from build123d import *

# Parameters (mm, degrees)
F0_W     = 17.78
F0_H     = 101.6
F0_R     = 2.794
F1_DEPTH = 5.08
F2_W     = 17.78
F2_H     = 12.7
F3_DEPTH = 19.05


with BuildPart() as f1:
    # F0 (on Top) → F1 (new body)
    with BuildSketch(Plane.XY):
        with Locations((0, 12.7)):
            Rectangle(F0_W, F0_H)
        with Locations((0, -30.513791)):
            Circle(F0_R, mode=Mode.SUBTRACT)
        with Locations((0, 20.286209)):
            Circle(F0_R, mode=Mode.SUBTRACT)
    extrude(amount=F1_DEPTH)

    # F2 (on face) → F3 (join)
    with BuildSketch(Plane.XY.offset(5.08)):
        with Locations((0, 57.15)):
            Rectangle(F2_W, F2_H)
    extrude(amount=F3_DEPTH)


solid = f1.part
Can you work these out from the model? Positions are in its coordinate system, mm. A direction names the side the tool comes from. Coordinates: 2 decimals unless noted, no trailing zeros. Write each loop counter-clockwise with the first axis right and the second up, starting at its lowest first coordinate (ties: lowest second). Pieces come first, ordered by that corner, then holes. Notation, with made-up numbers: (18, 73.25) - (58, 73.25) arc R18 cw to (58, 95.25) - close; hole circle Ø8 at (28.5, -21). An arc over 180 degrees is marked (long way). Return JSON: item names as keys, results as strings. Group by question number.
Item 1: Which directions (+Z, -Z, +X, -X, +Y, -Y) give clear straight access to the entire face, cutting with the end or side of a thin tool? Please do faces 5 (the face through (0, 7, 5.08)), 6 (the face through (-8.89, 24, 3)).
Item 2: If we section it at A-A (x = 0): Write out the boundary of the cut face in (y, z).
Item 3: I'm going to push flat-ended pins straight in: pin 1 Ø6 at (x, y) = (5.5, 28.5) entering from -Z; pin 2 Ø9 at (x, z) = (-0.5, 17) entering from -Y; pin 3 Ø3 at (x, y) = (-3, -13) entering from +Z. Where does each tip first touch, or does it pass through?
Item 4: If we section it at D-D (z = 9.5): Write out the boundary of the cut face in (x, y).
Item 5: We'd pull the mould along Y, two halves only. Please class faces 1 (the face through (0, 63.5, 12)), 2 (the face through (0, 57, 24.13)), 3 (the face through (-0.364, 23.056, 2.504)), 4 (the face through (-0.61, -33.24, 2.5)): pulls with the +Y half, pulls with the -Y half, needs draft (parallel to the pull), parting line crosses it, or undercut.
Item 6: If we section it at C-C (x = -7.5): Write out the boundary of the cut face in (y, z).
Item 7: If we section it at B-B (y = 19): Write out the boundary of the cut face in (x, z).
Item 8: Please list where these lines run through material, in increasing order: probe 1 along Y at (x, z) = (0, 4); probe 2 along Y at (x, z) = (-1.25, 3.5) (3 decimals); probe 3 along Y at (x, z) = (-6, 14.5).
Return value:
{
 "1": {"face 5": "+Z, +X, -X, -Y", "face 6": "+Z, -Z, -X, +Y, -Y"},
 "2": {"outline": "(-38.1, 0) - (-33.31, 0) - (-33.31, 5.08) - (-38.1, 5.08) - close; (-27.72, 0) - (17.49, 0) - (17.49, 5.08) - (-27.72, 5.08) - close; (23.08, 0) - (63.5, 0) - (63.5, 24.13) - (50.8, 24.13) - (50.8, 5.08) - (23.08, 5.08) - close"},
 "3": {"pin 1": "stops at z = 0", "pin 2": "stops at y = 50.8", "pin 3": "stops at z = 5.08"},
 "4": {"outline": "(-8.89, 50.8) - (8.89, 50.8) - (8.89, 63.5) - (-8.89, 63.5) - close"},
 "5": {"face 1": "pulls with the +Y half", "face 2": "needs draft", "face 3": "undercut", "face 4": "undercut"},
 "6": {"outline": "(-38.1, 0) - (63.5, 0) - (63.5, 24.13) - (50.8, 24.13) - (50.8, 5.08) - (-38.1, 5.08) - close"},
 "7": {"outline": "(-8.89, 0) - (-2.48, 0) - (-2.48, 5.08) - (-8.89, 5.08) - close; (2.48, 0) - (8.89, 0) - (8.89, 5.08) - (2.48, 5.08) - close"},
 "8": {"probe 1": "y = -38.1 to -33.31, -27.72 to 17.49, 23.08 to 63.5", "probe 2": "y = -38.1 to -33.013, -28.015 to 17.787, 22.785 to 63.5", "probe 3": "y = 50.8 to 63.5"}
}
